Could you check a few things on this drawing? It's one solid part, dimensions in mm from its lowest x, y, z. Give positions to 0.01 mm unless a question says otherwise; leave off trailing zeros. Write each loop counter-clockwise with the first axis right and the second up, starting at its lowest first coordinate (ties: lowest second). Pieces come first, ordered by that corner, then holes.
1. Suppose I cut it at D-D (x = 21). Please give me the cut outline in (y, z).
2. Suppose I cut it at B-B (x = 30). Please give me the cut outline in (y, z), and give its area (3 significant figures).
3. If I drill on probe 1 along Y at (x, z) = (32, 6.5); probe 2 along Z at (x, y) = (20, 22.5); probe 3 along Z at (x, y) = (29.5, 4.75) (1 decimal), over which ranges is the centre line in solid material (lowest first)?
4. Suppose I cut it at C-C (z = 21.5). Please give me the cut outline in (x, y) (1 decimal), and give its area (3 significant figures).
5. Suppose I cut it at A-A (y = 9.75). Please give me the cut outline in (x, z).
6. I'm going to push flat-ended pins straight in: pin 1 (1.5 mm diameter, centred on x = 25, y = 19, fed in from -Z) (1 decimal); pin 2 (4 mm diameter, centred on y = 17, z = 14.5, fed in from +X); pin 3 (10 mm diameter, centred on x = 9.5, z = 18, fed in from +Y); pin 4 (10.5 mm diameter, centred on x = 14, z = 10, fed in from +Y). Where does each tip first touch, or does it pass through?
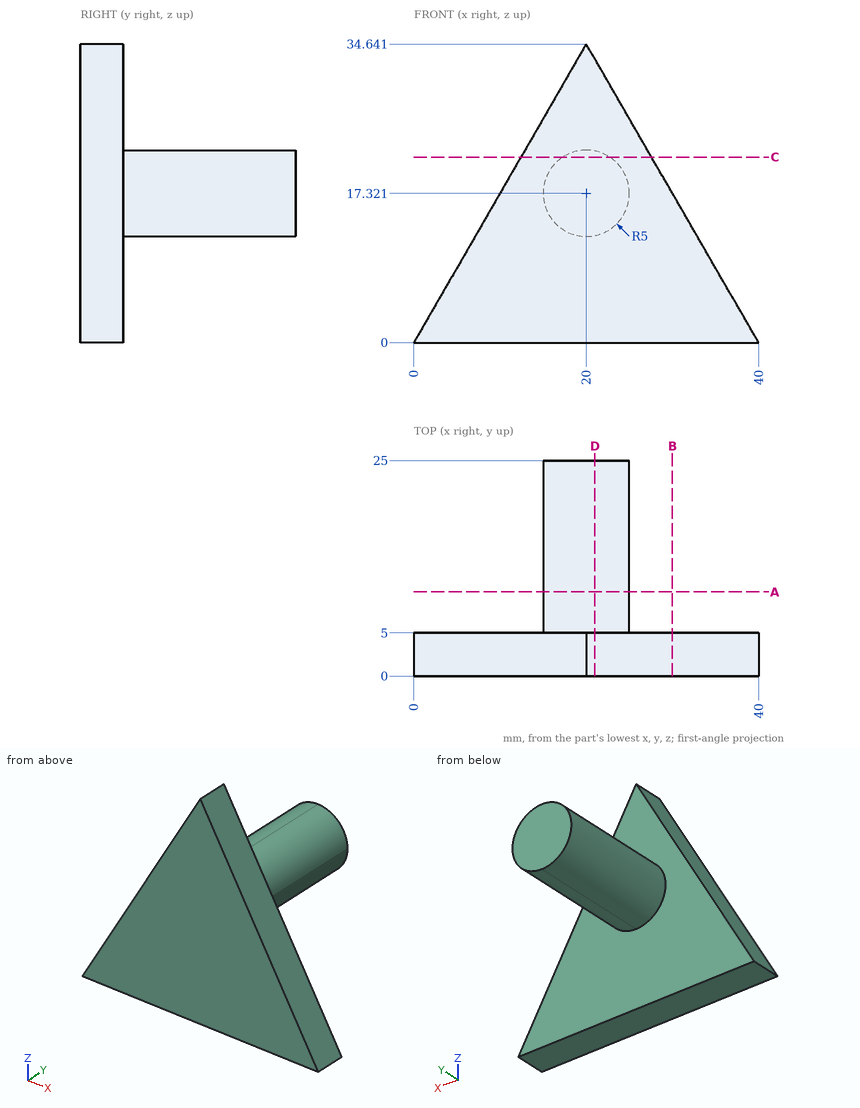
Checks:
1. outline: (0, 0) - (5, 0) - (5, 12.42) - (25, 12.42) - (25, 22.22) - (5, 22.22) - (5, 32.91) - (0, 32.91) - close
2. outline: (0, 0) - (5, 0) - (5, 17.32) - (0, 17.32) - close
2. area: 86.6 mm2
3. probe 1: y = 0 to 5
3. probe 2: z = 12.32 to 22.32
3. probe 3: z = 0 to 18.2
4. outline: (12.4, 0) - (27.6, 0) - (27.6, 5) - (22.7, 5) - (22.7, 25) - (17.3, 25) - (17.3, 5) - (12.4, 5) - close
4. area: 186 mm2
5. outline: circle Ø10 at (20, 17.32)
6. pin 1: stops at z = 14.7
6. pin 2: stops at x = 24.93
6. pin 3: stops at y = 5
6. pin 4: stops at y = 25
